Autodesk Inventor part; units mm, degrees
ref_plane "HOUSING_TO_DUMMY_XY" through (0, 0, 0) normal (0, 0, 1) x (1, 0, 0)
ref_plane "HOUSING_TO_DUMMY_YZ" through (0, 0, 0) normal (1, 0, 0) x (0, 1, 0)
ref_plane "HOUSING_TO_DUMMY_ZX" through (0, 0, 0) normal (0, 1, 0) x (0, 0, 1)
sketch "Sketch_1" plane through (0, 0, 0) normal (1, 0, 0) x (0, 0, -1)
  line L0 (-13, 15.1987) -> (-13, -15.1987)
  arc A0 (-13, -15.1987) -> (13, -15.1987) centre (0, 0) ccw
  line L1 (13, -15.1987) -> (13, 15.1987)
  arc A1 (13, 15.1987) -> (-13, 15.1987) centre (0, 0) ccw
extrude "Extrusion1" add sketch "Sketch_1" along normal mid plane 11
sketch "Sketch2" plane through (5.5, 0, 0) normal (1, 0, 0) x (0, 0, -1)
  point P0 (0, 0)
hole "Hole1" at (5.5, 0, 0) direction (-1, 0, 0) diameter 19 depth 11 counterbore diameter 22 counterbore depth 9
sketch "Sketch_9" plane through (0, 0, 0) normal (0, 0, 1) x (1, 0, 0)
  line L0 (3.65, 0) -> (2.5, 0)
  line L1 (2.5, 0) -> (2.5, 11.5)
  line L2 (2.5, 11.5) -> (3.65, 11.5)
  line L3 (3.65, 11.5) -> (3.65, 0)
  line L4 (3.65, 0) -> (2.5, 0)
revolve "Revolution1" cut sketch "Sketch_9" angle 360 about axis through (3.65, 0, 0) along (1, 0, 0)
sketch "Sketch_8" plane through (0, 0, 0) normal (0, 0, 1) x (1, 0, 0)
  line L0 (5.5, -15.5) -> (-5.5, -15.5)
  line L1 (-5.5, -15.5) -> (-5.5, -13)
  line L2 (-5.5, -13) -> (-5.067, -13.433)
  line L3 (-5.067, -13.433) -> (5.067, -13.433)
  line L4 (5.067, -13.433) -> (5.5, -13)
  line L5 (5.5, -13) -> (5.5, -15.5)
  line L6 (5.5, -15.5) -> (-5.5, -15.5)
revolve "Revolution2" cut sketch "Sketch_8" angle 360 about axis through (5.5, -15.5, 0) along (1, 0, 0)
thread "Thread1"
sketch "Sketch_2" plane through (0, 0, 0) normal (0, 0, 1) x (1, 0, 0)
  line L0 (5.5, 15.5) -> (-5.5, 15.5)
  line L1 (-5.5, 15.5) -> (-5.5, 18)
  line L2 (-5.5, 18) -> (-5.067, 17.567)
  line L3 (-5.067, 17.567) -> (5.067, 17.567)
  line L4 (5.067, 17.567) -> (5.5, 18)
  line L5 (5.5, 18) -> (5.5, 15.5)
  line L6 (5.5, 15.5) -> (-5.5, 15.5)
revolve "Revolution3" cut sketch "Sketch_2" angle 360 about axis through (5.5, 15.5, 0) along (1, 0, 0)
thread "Thread2"
ref_plane "HOUSING_TO_DUMMY_XY" through (0, 0, 0) normal (0, 0, 1) x (1, 0, 0)
ref_plane "HOUSING_TO_DUMMY_YZ" through (0, 0, 0) normal (1, 0, 0) x (0, 1, 0)
ref_plane "HOUSING_TO_DUMMY_ZX" through (0, 0, 0) normal (0, 1, 0) x (0, 0, 1)
ref_plane "bgcab_to_rring_XY" through (2.5, 0, 0) normal (-1, 0, 0) x (0, 0, -1)
ref_plane "bgcab_to_rring_YZ" through (2.5, 0, 0) normal (0, 0, -1) x (0, -1, 0)
ref_plane "bgcab_to_rring_ZX" through (2.5, 0, 0) normal (0, -1, 0) x (-1, 0, 0)
ref_plane "to_bearings_XY" through (-3.5, 0, 0) normal (-1, 0, 0) x (0, 0, -1)
ref_plane "to_bearings_YZ" through (-3.5, 0, 0) normal (0, 0, -1) x (0, -1, 0)
ref_plane "to_bearings_ZX" through (-3.5, 0, 0) normal (0, -1, 0) x (-1, 0, 0)
properties part number "BGTAB6900VV_h"
Part model, mm, in its own coordinate system. A direction names the side the tool comes from. Give positions to 0.01 mm unless a question says otherwise; leave off trailing zeros. Order: outer loops, then holes, each group sorted by start corner. A loop starts at its lowest first (then second) coordinate and runs counter-clockwise, first axis right, second up. Notation, with made-up numbers: M 22.5,37 L 55.5,37 A24 ccw 55.5,49 Z; hole C -34,-2.75 d7. An arc over 180 degrees is marked long. Use a Markdown table: item, result. Add a question column.
(1) Saw through at C-C, the plane z = -4.5. Give the cut face in (x, y).
(2) Saw through at A-A, the plane x = -4. Give the cut face in (y, z), and give its area (3 significant figures).
(3) 3-axis set-ups, long thin cutter, end or side, ignore diameter. For faces 4 (the face through (4.56, 10.74, 2.38)), 5 (the face through (3.1, -1.5, 11.4)), 6 (the face through (0, -20, 0)): which of +Z, -Z, +X, -X, +Y, -Y reach the whole face in a straight line?
(4) Drop flat-ended pins along their axis: P1, Ø6, axis at x = 0.5, z = 8, coming from the +Y side; P2, Ø13, axis at y = 0, z = 0, coming from the -X side. Give the stop position or say it passes through.
(5) Mould opens along Z. For faces 1 (the face through (0, 0, 13)), 2 (the face through (-5.5, 9.2, 3.1)), 3 (the face through (-3.5, 0, 10)) say: +Z half, -Z half, draft (parallel to the pull), parting line (faces both ways), or undercut.
(6) Saw through at B-B, the plane y = 0. Give the cut face in (x, z), and give its area (4 significant figures).
(7) Saw through at D-D, the plane z = 0. Give the number of separate pieces and of enclosed holes in the cut face, and give its area (3 significant figures).
(8) Probe line 1 along Y through (x, z) = (2.75, 1) (3 decimals); line 2 along Z through (x, y) = (0, 0.5); line 3 along X through (y, z) = (9, -7). List the from-to ranges inside material, lowest first. Write a range as [from, to].
Answer key:
| question | item | result |
|---|---|---|
| 1 | outline | M -5.5,-19.49 L 5.5,-19.49 L 5.5,-10.04 L 3.65,-10.04 L 3.65,-10.58 L 2.5,-10.58 L 2.5,-10.04 L -3.5,-10.04 L -3.5,-8.37 L -5.5,-8.37 Z; M -5.5,8.37 L -3.5,8.37 L -3.5,10.04 L 2.5,10.04 L 2.5,10.58 L 3.65,10.58 L 3.65,10.04 L 5.5,10.04 L 5.5,19.49 L -5.5,19.49 Z |
| 2 | outline | M -15.2,-13 L 15.2,-13 A20 ccw 15.2,13 L -15.2,13 A20 ccw Z; hole C -15.5,0 d4.13; hole C 0,0 d19; hole C 15.5,0 d4.13 |
| 2 | area | 651 mm^2 |
| 3 | face 4 | +X |
| 3 | face 5 | none |
| 3 | face 6 | +X, -X, -Y |
| 4 | P1 | y = 19.36 |
| 4 | P2 | through |
| 5 | face 1 | +Z half |
| 5 | face 2 | draft |
| 5 | face 3 | undercut |
| 6 | outline | M -5.5,-13 L 5.5,-13 L 5.5,-11 L 3.65,-11 L 3.65,-11.5 L 2.5,-11.5 L 2.5,-11 L -3.5,-11 L -3.5,-9.5 L -5.5,-9.5 Z; M -5.5,9.5 L -3.5,9.5 L -3.5,11 L 2.5,11 L 2.5,11.5 L 3.65,11.5 L 3.65,11 L 5.5,11 L 5.5,13 L -5.5,13 Z |
| 6 | area | 48.85 mm^2 |
| 7 | separate pieces | 4 |
| 7 | enclosed holes | 0 |
| 7 | area | 111 mm^2 |
| 8 | line 1 | [-19.975, -17.309], [-13.691, -11.456], [11.456, 13.691], [17.309, 19.975] |
| 8 | line 2 | [-13, -10.99], [10.99, 13] |
| 8 | line 3 | [-5.5, 2.5], [3.65, 5.5] |
